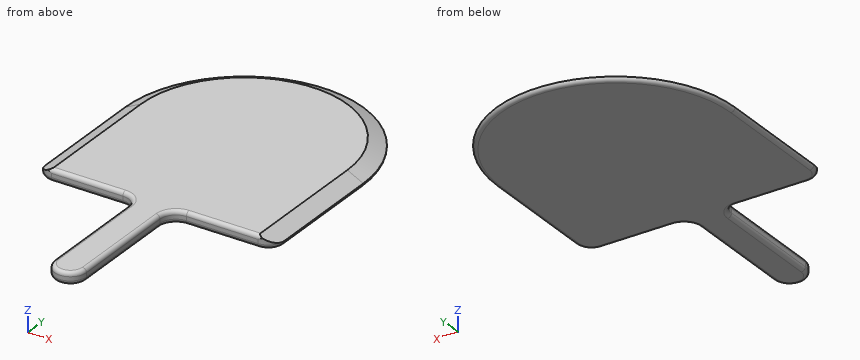
from build123d import *

# Parameters (mm, degrees)
F1_DEPTH    = 19.05
F2_T1_DEPTH = 256.2816533942
F2_T4_ANGLE = 180
F3_R        = 6.35
F4_R        = 6.34999


# Not quite as in the source:
# - a fillet or chamfer that OpenCascade refuses, or shapes differently, is made with other operations: its cross-section is extruded or revolved along the edge and cut away or added
# - a fillet or chamfer is up to 0.001 mm smaller than in the source, because OpenCascade refuses the exact size


with BuildPart() as f1:
    # F0 (on Top) → F1 (new body)
    with BuildSketch(Plane.XY):
        with BuildLine():
            Line((190.5, -190.5), (190.5, 0))
            ThreePointArc((190.5, 0), (0, 190.5), (-190.5, 0))
            Line((-190.5, 0), (-190.5, -190.5))
            ThreePointArc((-190.5, -190.5), (-183.0605122421, -208.4605122421), (-165.1, -215.9))
            Line((-165.1, -215.9), (-50.8, -215.9))
            ThreePointArc((-50.8, -215.9), (-32.8394877579, -223.3394877579), (-25.4, -241.3))
            Line((-25.4, -241.3), (-25.4, -419.1))
            ThreePointArc((-25.4, -419.1), (0, -444.5), (25.4, -419.1))
            Line((25.4, -419.1), (25.4, -241.3))
            ThreePointArc((25.4, -241.3), (32.8394877579, -223.3394877579), (50.8, -215.9))
            Line((50.8, -215.9), (165.1, -215.9))
            ThreePointArc((165.1, -215.9), (183.0605122421, -208.4605122421), (190.5, -190.5))
        make_face()
    extrude(amount=F1_DEPTH)

    # F2: chamfer of 12.7 x 25.4 on 3 edges, made by hand

    # F2_s2 → F2_t1 (cut)
    with BuildSketch(Plane.XZ):
        Polygon((-190.5, 6.35), (-165.1, 19.05), (-190.5, 19.05), align=None)
        Polygon((190.5, 6.35), (165.1, 19.05), (190.5, 19.05), align=None)
    extrude(amount=F2_T1_DEPTH, mode=Mode.SUBTRACT)

    # F2_s3 → F2_t4 (revolve, cut)
    with BuildSketch(Plane.XZ):
        Polygon((190.5, 6.35), (165.1, 19.05), (190.5, 19.05), align=None)
    revolve(axis=Axis((0, 0, 19.05), (0, 0, 1)), revolution_arc=F2_T4_ANGLE, mode=Mode.SUBTRACT)

    # F3
    f3_edges = [f1.edges().sort_by_distance(p)[0] for p in [
        (0, -444.5, 19.05),
    ]]
    fillet(f3_edges, radius=F3_R)

    # F4 (radius 6.35 in the source; OpenCascade refuses exactly that, so slightly less here)
    f4_edges = [f1.edges().sort_by_distance(p)[0] for p in [
        (25.4, -330.2, 0),
        (32.839488, -223.339488, 0),
        (107.95, -215.9, 0),
        (183.060512, -208.460512, 0),
        (190.5, -95.25, 0),
        (0, 190.5, 0),
        (-190.5, -95.25, 0),
        (-183.060512, -208.460512, 0),
        (-107.95, -215.9, 0),
        (-32.839488, -223.339488, 0),
        (-25.4, -330.2, 0),
        (0, -444.5, 0),
    ]]
    fillet(f4_edges, radius=F4_R)


solid = f1.part
Here's how the part is built. I have some questions about the finished solid (model axes, mm). Coordinates: 2 decimals unless noted, no trailing zeros. Order: outer loops, then holes, each group sorted by start corner. A loop starts at its lowest first (then second) coordinate and runs counter-clockwise, first axis right, second up. Notation, with made-up numbers: (-32.75, 85) -> (-21.75, 85) arc R27 ccw to (-21.75, 103) -> close; hole circle Ø4 at (9, 82.25). An arc over 180 degrees is marked (long way). Answer in a Markdown table with one row per item.
(1) Please list where these lines run through material, in increasing order: probe 1 along X at (y, z) = (-295, 11.5); probe 2 along Y at (x, z) = (41, 3.75); probe 3 along Y at (x, z) = (-13, 11.25).
Answer key:
| item | result |
|---|---|
| probe 1 | -25.4 to 25.4 |
| probe 2 | -217.26 to 185.47 |
| probe 3 | -440.92 to 180.23 |
(2) Will these pins go through, and if not, where does the flat tip stop? pin 1 Ø1.5 at (y, z) = (-187, 3.5) entering from +X; pin 2 Ø3 at (x, z) = (-90.5, 9.5) entering from -Y; pin 3 Ø3 at (y, z) = (-295, 10.5) entering from -X.
Answer key:
| item | result |
|---|---|
| pin 1 | x = 190.14 |
| pin 2 | y = -215.9 |
| pin 3 | x = -25.4 |
(3) I want a section at B-B on y = -292.5. List the corners of the cut face in (x, z) for me, then the cut area to 3 significant figures.
Answer key:
| item | result |
|---|---|
| outline | (-25.4, 6.35) arc R6.35 ccw to (-19.05, 0) -> (19.05, 0) arc R6.35 ccw to (25.4, 6.35) -> (25.4, 12.7) arc R6.35 ccw to (19.05, 19.05) -> (-19.05, 19.05) arc R6.35 ccw to (-25.4, 12.7) -> close |
| area | 933 mm^2 |
